Design review of the part shown in the three views and the two pictorial views. Dimensions are in mm from the part's minimum x, y and z. Round coordinates to 2 decimals unless told otherwise and drop trailing zeros. Order: outer loops, then holes, each group sorted by start corner. A loop starts at its lowest first (then second) coordinate and runs counter-clockwise, first axis right, second up.
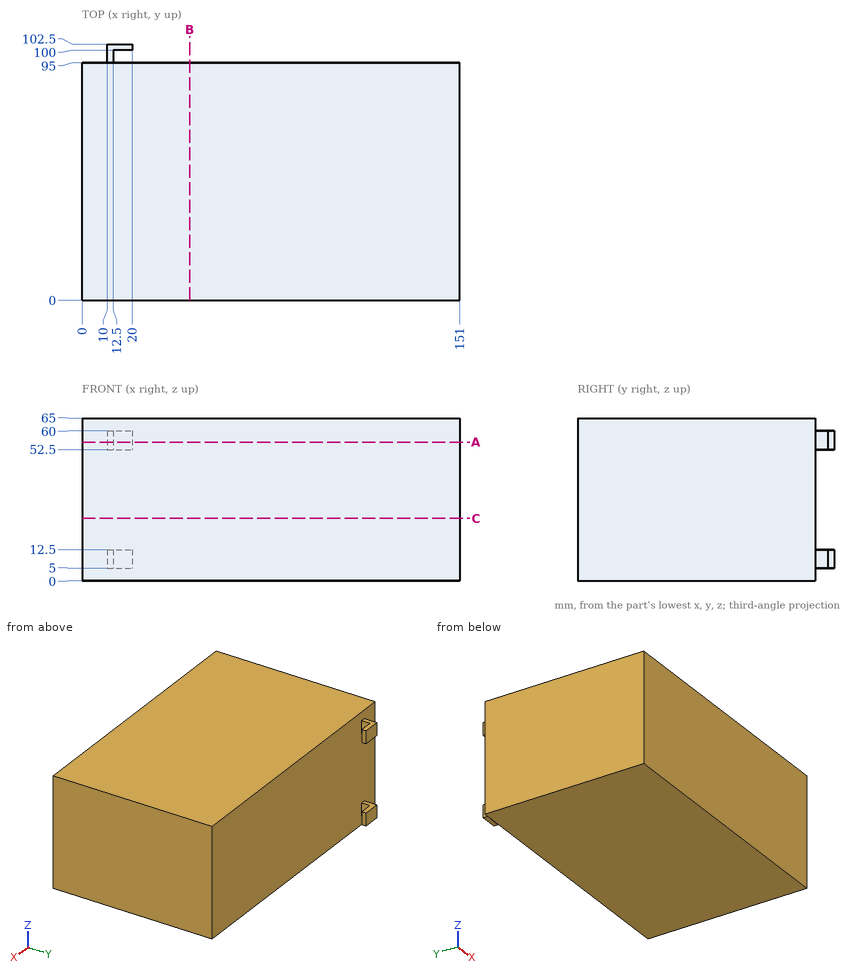
(1) Insertion check: pin 1 (1.5 mm diameter, centred on y = 97.5, z = 57, fed in from +X); pin 2 (4 mm diameter, centred on x = 16, y = 97.5, fed in from +Z); pin 3 (2 mm diameter, centred on y = 101.5, z = 7, fed in from +X); pin 4 (4 mm diameter, centred on x = 13.5, y = 99, fed in from -Z). Each pin has a flat end and moves straight along its axis. Give the tip position at first contact, or say it passes through.
Data:
pin 1: stops at x = 12.5
pin 2: passes through
pin 3: stops at x = 20
pin 4: stops at z = 5
(2) Consider section A-A (z = 55.5). Write out the cut boundary in (x, y).
Data:
outline: (0, 0) - (151, 0) - (151, 95) - (12.5, 95) - (12.5, 100) - (20, 100) - (20, 102.5) - (10, 102.5) - (10, 95) - (0, 95) - close
(3) To check wall thickness, follow probe 1 along Y at (x, z) = (39.5, 32). State the ranges of the line that lie inside material, in increasing order.
Data:
probe 1: y = 0 to 95
(4) Consider section C-C (z = 25). Write out the cut boundary in (x, y), and give its area (3 significant figures).
Data:
outline: (0, 0) - (151, 0) - (151, 95) - (0, 95) - close
area: 14,300 mm2
(5) Consider section B-B (x = 43). Write out the cut boundary in (y, z).
Data:
outline: (0, 0) - (95, 0) - (95, 65) - (0, 65) - close
